```python
from build123d import *

# Parameters (mm, degrees)
SKETCH5_R               = 16
BOSS_EXTRUDE3_DEPTH     = 3
SKETCH6_R               = 9.5
BOSS_EXTRUDE4_DEPTH     = 10
SKETCH7_R               = 7
CUT_EXTRUDE1_DEPTH      = 27.095976701
SKETCH8_R               = 2
CUT_EXTRUDE2_DEPTH      = 27.095976701
CUT_EXTRUDE4_DEPTH      = 27.095976701
CUT_EXTRUDE4_DEPTH_BACK = 27.095976701
SKETCH9_R               = 2
FILLET1_R               = 0.5


with BuildPart() as part:
    # Sketch5 → Boss-Extrude3 (new body)
    with BuildSketch(Plane.XY):
        Circle(SKETCH5_R)
    extrude(amount=BOSS_EXTRUDE3_DEPTH)

    # Sketch6 → Boss-Extrude4 (add)
    with BuildSketch(Plane.XY.offset(3)):
        Circle(SKETCH6_R)
    extrude(amount=BOSS_EXTRUDE4_DEPTH)

    # Sketch7 → Cut-Extrude1 (cut, through all)
    with BuildSketch(Plane.XY.offset(13)):
        Circle(SKETCH7_R)
    extrude(amount=-CUT_EXTRUDE1_DEPTH, mode=Mode.SUBTRACT)

    # Sketch8 → Cut-Extrude2 (cut, through all)
    with BuildSketch(Plane(origin=(0, 0, 0), x_dir=(-1, 0, 0), z_dir=(0, 0, -1))):
        with Locations((12, 0)):
            Circle(SKETCH8_R)
        with Locations((0, -12)):
            Circle(SKETCH8_R)
        with Locations((-12, 0)):
            Circle(SKETCH8_R)
        with Locations((0, 12)):
            Circle(SKETCH8_R)
    extrude(amount=-CUT_EXTRUDE2_DEPTH, mode=Mode.SUBTRACT)

    # Sketch9 → Cut-Extrude4 (cut, two sides: drawn at the far end of the back side and taken through both)
    with BuildSketch(Plane(origin=(0, 0, 0), x_dir=(1, 0, 0), z_dir=(0, 1, 0)).offset(-CUT_EXTRUDE4_DEPTH_BACK)):
        with Locations(Location((0, -8, 0), (0, 0, 270))):
            Circle(SKETCH9_R)
    extrude(amount=CUT_EXTRUDE4_DEPTH + CUT_EXTRUDE4_DEPTH_BACK, mode=Mode.SUBTRACT)

    # Fillet1
    fillet1_edges = [part.edges().sort_by_distance(p)[0] for p in [
        (-9.5, 0, 13),
    ]]
    fillet(fillet1_edges, radius=FILLET1_R)


solid = part.part
```
CAD build for the part. Positions are in the model's coordinates, mm. A direction names the side the tool comes from. Coordinates: 2 decimals unless noted, no trailing zeros. Order: outer loops, then holes, each group sorted by start corner. A loop starts at its lowest first (then second) coordinate and runs counter-clockwise, first axis right, second up. Notation, with made-up numbers: (-2, -2.5) - (19, -2.5) arc R18 cw to (19, 27.5) - close; hole circle Ø8 at (59, 30). An arc over 180 degrees is marked (long way). Answer in a Markdown table with one row per item.
1. Drill centre lines: L1, parallel to Z at x = 0, y = -8.45; L2, parallel to Z at x = -2, y = -10; L3, parallel to Y at x = 0, z = 4. Where is each one in solid material? Low to high. Write a range as from..to.
Answer:
| item | result |
|---|---|
| L1 | 0..6, 10..13 |
| L2 | 0..3 |
| L3 | -9.5..-7, 7..9.5 |
2. 3-axis set-ups, long thin cutter, end or side, ignore diameter. For faces 1 (the face through (13.6, -1.2, 1.5)), 2 (the face through (7, -7, 3)): which of +Z, -Z, +X, -X, +Y, -Y reach the whole face in a straight line?
Answer:
| item | result |
|---|---|
| face 1 | +Z, -Z |
| face 2 | +Z |
3. Slice it at B-B, the plane x = -12. List the corners of the cut face in (y, z).
Answer:
| item | result |
|---|---|
| outline | (-10.58, 0) - (-2, 0) - (-2, 3) - (-10.58, 3) - close; (2, 0) - (10.58, 0) - (10.58, 3) - (2, 3) - close |
4. Slice it at A-A, the plane x = 0. Give the number of separate pieces and of enclosed holes in the cut face, then the cut area to 3 significant figures.
Answer:
| item | result |
|---|---|
| separate pieces | 6 |
| enclosed holes | 0 |
| area | 59.9 mm² |
5. Pull direction Y, two halves, no side cores. Call faces 3 (the face through (0, -10, 1)), 4 (the face through (-3.47, -15.62, 1.48)), 5 (the face through (7, -3, 0)): +Y half, -Y half, draft (parallel to the pull), parting line (faces both ways), or undercut.
Answer:
| item | result |
|---|---|
| face 3 | undercut |
| face 4 | parting line |
| face 5 | draft |
6. Flat gauge pins, fed straight in: P1, Ø4.5, axis at x = 0, z = 8, coming from the -Y side; P2, Ø2.5, axis at x = -12, y = 0, coming from the +Z side; P3, Ø5, axis at y = -9, z = 6.5, coming from the +X side; P4, Ø1, axis at y = -4.5, z = 1.5, coming from the -X side. Where does each tip first touch, or does it go through?
Answer:
| item | result |
|---|---|
| P1 | y = -9.5 |
| P2 | through |
| P3 | x = 6.93 |
| P4 | x = -15.49 |
